from build123d import *

# Parameters (mm, degrees)
SKETCH_R        = 1.75
PAD_DEPTH       = 2
PAD001_DEPTH    = 5
SKETCH002_W     = 53
SKETCH002_H     = 81
PAD002_DEPTH    = 2
SKETCH003_W     = 53
SKETCH003_H     = 81
SKETCH003_W_2   = 49
SKETCH003_H_2   = 77
PAD003_DEPTH    = 49.5
PAD004_DEPTH    = 2
SKETCH005_W     = 43
SKETCH005_H     = 43.5
POCKET_DEPTH    = 81
SKETCH006_W     = 71
SKETCH006_H     = 43.5
POCKET001_DEPTH = 2
SKETCH007_W     = 77
SKETCH007_H     = 49.5
POCKET002_DEPTH = 5


with BuildPart() as part:
    # Sketch → Pad (new body)
    with BuildSketch(Plane.XY):
        Polygon((-13.279056, 21), (-13.279056, -21), (-11.547005, -22), (24.826062, -1), (24.826062, 1), (-11.547005, 22), align=None)
        with Locations((-7.279056, 0)):
            Circle(SKETCH_R, mode=Mode.SUBTRACT)
        with Locations((3.639528, 6.303848)):
            Circle(SKETCH_R, mode=Mode.SUBTRACT)
        with Locations((3.639528, -6.303848)):
            Circle(SKETCH_R, mode=Mode.SUBTRACT)
        Polygon((6.558112, 0), (-3.279056, 5.679492), (-3.279056, -5.679492), align=None, mode=Mode.SUBTRACT)
    extrude(amount=PAD_DEPTH)

    # Sketch001 (on Face14 of Pad) → Pad001 (join)
    with BuildSketch(Plane.XY.offset(2)):
        Polygon((-13.279056, 21), (-11.547005, 22), (24.826062, 1), (24.826062, -1), (-11.547005, -22), (-13.279056, -21), align=None)
        Polygon((22.558112, 0), (-11.279056, 19.535898), (-11.279056, -19.535898), align=None, mode=Mode.SUBTRACT)
    extrude(amount=PAD001_DEPTH)

    # Sketch002 (on Face17 of Pad001) → Pad002 (join)
    with BuildSketch(Plane.XY.offset(7)):
        with Locations((3.5, 0)):
            Rectangle(SKETCH002_W, SKETCH002_H)
        Polygon((-11.279056, 19.535898), (22.558112, 0), (-11.279056, -19.535898), align=None, mode=Mode.SUBTRACT)
    extrude(amount=PAD002_DEPTH)

    # Sketch003 (on Face29 of Pad002) → Pad003 (join)
    with BuildSketch(Plane.XY.offset(9)):
        with Locations((3.5, 0)):
            Rectangle(SKETCH003_W, SKETCH003_H)
        with Locations((3.5, 0)):
            Rectangle(SKETCH003_W_2, SKETCH003_H_2, mode=Mode.SUBTRACT)
    extrude(amount=PAD003_DEPTH)

    # Sketch004 (on Face36 of Pad003) → Pad004 (join)
    with BuildSketch(Plane.XY.offset(58.5)):
        Polygon((-23, 40.5), (30, 40.5), (30, 34.25), (-19, 34.25), (-19, -34.25), (30, -34.25), (30, -40.5), (-23, -40.5), align=None)
    extrude(amount=PAD004_DEPTH)

    # Sketch005 (on Face32 of Pad004) → Pocket (cut)
    with BuildSketch(Plane.XZ.offset(40.5)):
        with Locations((3.5, 33.75)):
            Rectangle(SKETCH005_W, SKETCH005_H)
    extrude(amount=-POCKET_DEPTH, mode=Mode.SUBTRACT)

    # Sketch006 (on Face30 of Pocket) → Pocket001 (cut)
    with BuildSketch(Plane(origin=(-23, 0, 0), x_dir=(0, -1, 0), z_dir=(-1, 0, 0))):
        with Locations((0, 33.75)):
            Rectangle(SKETCH006_W, SKETCH006_H)
    extrude(amount=-POCKET001_DEPTH, mode=Mode.SUBTRACT)

    # Sketch007 (on Face31 of Pocket001) → Pocket002 (cut)
    with BuildSketch(Plane.YZ.offset(30)):
        with Locations((0, 33.75)):
            Rectangle(SKETCH007_W, SKETCH007_H)
    extrude(amount=-POCKET002_DEPTH, mode=Mode.SUBTRACT)


solid = part.part
Verification items for the finished model (mm, model axes). A direction names the side the tool comes from. Give positions to 0.01 mm unless a question says otherwise; leave off trailing zeros. Loops run counter-clockwise (first coordinate to the right, second up) from the corner with the lowest first, then second, coordinate; pieces in that order, holes last. Notation, with made-up numbers: (87, 15.5) - (116, 15.5) arc R23 cw to (116, 32.5) - close; hole circle Ø7 at (25, -27.5). An arc over 180 degrees is marked (long way). Write item = value, one per line. Start each with the question number.
Q1. Thickness scan on line 1 (Z direction, x = -19, y = 35); line 2 (Y direction, x = 9, z = 57); line 3 (Z direction, x = -14, y = -1). Record the ranges inside material, lowest first.
Q2. Depth check by flat-ended pin: P1, Ø10, axis at x = 6.5, y = 23.5, coming from the -Z side; P2, Ø1, axis at y = -0.5, z = 2, coming from the +X side; P3, Ø1.6, axis at y = -10, z = 59, coming from the +X side. Enter the tip coordinate at first touch or a pass-through.
Q3. Cross-section at A-A, the plane z = 31. Enter the section's corners in (x, y), and give its area (3 significant figures).
Q4. Mould release check, pull along Y, two halves, no side actions. Record for faces 5 (the face through (25, -40, 33)), 6 (the face through (5, -34.25, 59)), 7 (the face through (-12.401, -21.507, 3.451)): released by +Y, released by -Y, zero draft, split by the parting line, or undercut.
Q5. Cross-section at B-B, the plane z = 5. Enter the section's corners in (x, y), and give its area (3 significant figures).
Q6. Cross-section at D-D, the plane y = -26. Enter the section's corners in (x, z), and give its area (3 significant figures).
Q7. Cross-section at C-C, the plane x = 12.5. Enter the section's corners in (y, z).
Q8. Tool access check on faces 1 (the face through (3, -40, 12)), 2 (the face through (5, -38.5, 56)), 3 (the face through (-19, 0, 59)), 4 (the face through (2, 5, 2)). Record the directions out of +Z, -Z, +X, -X, +Y, -Y that give a thin tool (end or side, any length) a straight path to the whole face; none if there is none.
Answer key:
q1.line_1 = 7 to 9, 58.5 to 60.5
q1.line_2 = -40.5 to -38.5, 38.5 to 40.5
q1.line_3 = 7 to 9
q2.P1 = 7
q2.P2 = 24.83
q2.P3 = -19
q3.outline = (-23, -40.5) - (-18, -40.5) - (-18, -38.5) - (-21, -38.5) - (-21, -35.5) - (-23, -35.5) - close; (-23, 35.5) - (-21, 35.5) - (-21, 38.5) - (-18, 38.5) - (-18, 40.5) - (-23, 40.5) - close; (25, -40.5) - (30, -40.5) - (30, -38.5) - (25, -38.5) - close; (25, 38.5) - (30, 38.5) - (30, 40.5) - (25, 40.5) - close
q3.area = 52.0 mm^2
q4.face_5 = zero draft
q4.face_6 = undercut
q4.face_7 = released by -Y
q5.outline = (-13.28, -21) - (-11.55, -22) - (24.83, -1) - (24.83, 1) - (-11.55, 22) - (-13.28, 21) - close; hole (-11.28, -19.54) - (22.56, 0) - (-11.28, 19.54) - close
q5.area = 250 mm^2
q6.outline = (-23, 7) - (30, 7) - (30, 9) - (-21, 9) - (-21, 12) - (-23, 12) - close; (-23, 55.5) - (-21, 55.5) - (-21, 58.5) - (-19, 58.5) - (-19, 60.5) - (-23, 60.5) - close
q6.area = 126 mm^2
q7.outline = (-40.5, 7) - (-8.12, 7) - (-8.12, 0) - (8.12, 0) - (8.12, 7) - (40.5, 7) - (40.5, 12) - (38.5, 12) - (38.5, 9) - (5.81, 9) - (5.81, 2) - (-5.81, 2) - (-5.81, 9) - (-38.5, 9) - (-38.5, 12) - (-40.5, 12) - close; (-40.5, 55.5) - (-38.5, 55.5) - (-38.5, 58.5) - (-34.25, 58.5) - (-34.25, 60.5) - (-40.5, 60.5) - close; (34.25, 58.5) - (38.5, 58.5) - (38.5, 55.5) - (40.5, 55.5) - (40.5, 60.5) - (34.25, 60.5) - close
q8.face_1 = +Y, -Y
q8.face_2 = +X
q8.face_3 = +Z, +X
q8.face_4 = +Z
